Check sheet for the modelled part. Datum: model origin and axes. Units: mm. Face numbers are marked on the shaded views. A direction names the side the tool comes from. Give positions to 0.01 mm unless a question says otherwise; leave off trailing zeros. Loops run counter-clockwise (first coordinate to the right, second up) from the corner with the lowest first, then second, coordinate; pieces in that order, holes last. Notation, with made-up numbers: (87, 47.5) -> (97, 47.5) arc R31 cw to (97, 72.5) -> close; hole circle Ø1 at (68.5, 71.5). An arc over 180 degrees is marked (long way). Answer as CSV lines item,"result". Start each with the question number.
(1) Section check A-A on y = 0. Enter the section's corners in (x, z) (3 decimals).
(2) Material ranges on line 1 (Z direction, x = -11.5, y = -8.5); line 2 (Z direction, x = 3.5, y = -14); line 3 (X direction, y = -12, z = -45), recorded low to high. Write a range as from..to.
(3) Access from +Z, -Z, +X, -X, +Y, -Y to the whole of each face (thin tool, end or side, straight path). Record for the marked faces 1 and 2.
(4) Section check D-D on z = 29. Enter the section's corners in (x, y).
(5) Section check B-B on z = -72. Enter the section's corners in (x, y) (3 decimals).
(6) Gauge pin test, flat ends, axial feed: pin 1 Ø2 at (y, z) = (-15.5, -110) entering from -X; pin 2 Ø12 at (y, z) = (-11, 16.5) entering from -X; pin 3 Ø1.6 at (x, y) = (0, 7) entering from +Z. Record the tip position at first contact, or that the pin passes through.
(7) Section check C-C on x = 15.5. Enter the section's corners in (y, z).
from build123d import *

# Parameters (mm, degrees)
BOSS_EXTRUDE1_DEPTH = 15
SKETCH2_R           = 20.775
BOSS_EXTRUDE2_DEPTH = 5
SKETCH3_R           = 9.525
BOSS_EXTRUDE3_DEPTH = 127
SKETCH6_R           = 6
BOSS_EXTRUDE5_DEPTH = 50


with BuildPart() as part:
    # Sketch1 → Boss-Extrude1 (new body)
    with BuildSketch(Plane.XY):
        with BuildLine():
            Line((-2, 7.7), (2, 7.7))
            Line((2, 7.7), (2, 5.656854249))
            ThreePointArc((2, 5.656854249), (0, -6), (-2, 5.656854249))
            Line((-2, 5.656854249), (-2, 7.7))
        make_face()
    extrude(amount=BOSS_EXTRUDE1_DEPTH)

    # Sketch2 → Boss-Extrude2 (add)
    with BuildSketch(Plane(origin=(0, 0, 0), x_dir=(-1, 0, 0), z_dir=(0, 0, -1))):
        Circle(SKETCH2_R)
    extrude(amount=BOSS_EXTRUDE2_DEPTH)

    # Sketch3 → Boss-Extrude3 (add)
    with BuildSketch(Plane(origin=(0, 0, -5), x_dir=(-1, 0, 0), z_dir=(0, 0, -1))):
        with Locations((0, -11.25)):
            Circle(SKETCH3_R)
    extrude(amount=BOSS_EXTRUDE3_DEPTH)

    # Sketch6 → Boss-Extrude5 (add)
    with BuildSketch(Plane.XY.offset(15)):
        Circle(SKETCH6_R)
    extrude(amount=BOSS_EXTRUDE5_DEPTH)


solid = part.part
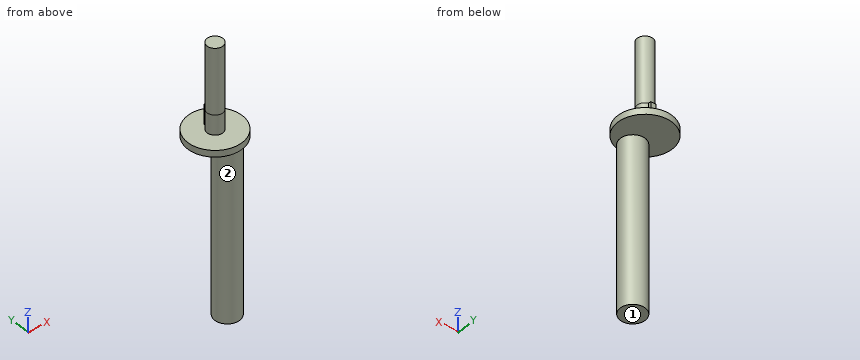
Working result:
1,outline,"(-20.775, -5) -> (20.775, -5) -> (20.775, 0) -> (6, 0) -> (6, 65) -> (-6, 65) -> (-6, 0) -> (-20.775, 0) -> close"
2,line 1,"z = -5..0"
2,line 2,"z = -132..0"
2,line 3,"x = -9.5..9.5"
3,face 1,"-Z, +X, -X, +Y, -Y"
3,face 2,"-Z"
4,outline,"circle Ø12 at (0, 0)"
5,outline,"circle Ø19.05 at (0, -11.25)"
6,pin 1,"stops at x = -8.95"
6,pin 2,"stops at x = -3.32"
6,pin 3,"stops at z = 15"
7,outline,"(-13.83, -5) -> (13.83, -5) -> (13.83, 0) -> (-13.83, 0) -> close"
